Input: dimensioned drawing with shaded views. Units: mm. Origin: part minimum x, y, z. Round coordinates to 2 decimals unless told otherwise and drop trailing zeros. Order: outer loops, then holes, each group sorted by start corner. A loop starts at its lowest first (then second) coordinate and runs counter-clockwise, first axis right, second up. Notation, with made-up numbers: M -9,10 L 32,10 A10 ccw 32,27 Z; hole C -34.5,-18.5 d9. An arc over 180 degrees is marked long. Use one line per item in the form item = value. Start each with the question number.
Q1. Material intervals for probe 1 along Y at (x, z) = (128.5, 2.45); probe 2 along X at (y, z) = (38, 1.25); probe 3 along X at (y, z) = (9, 2.2), sorted ascending.
Q2. Section B-B (x = 63). Return the cut outline in (y, z).
Q3. Section C-C (z = 1.1). Return the cut outline in (x, y).
Q4. Section A-A (y = 65.5). Return the cut outline in (x, z), plus the area to 3 significant figures.
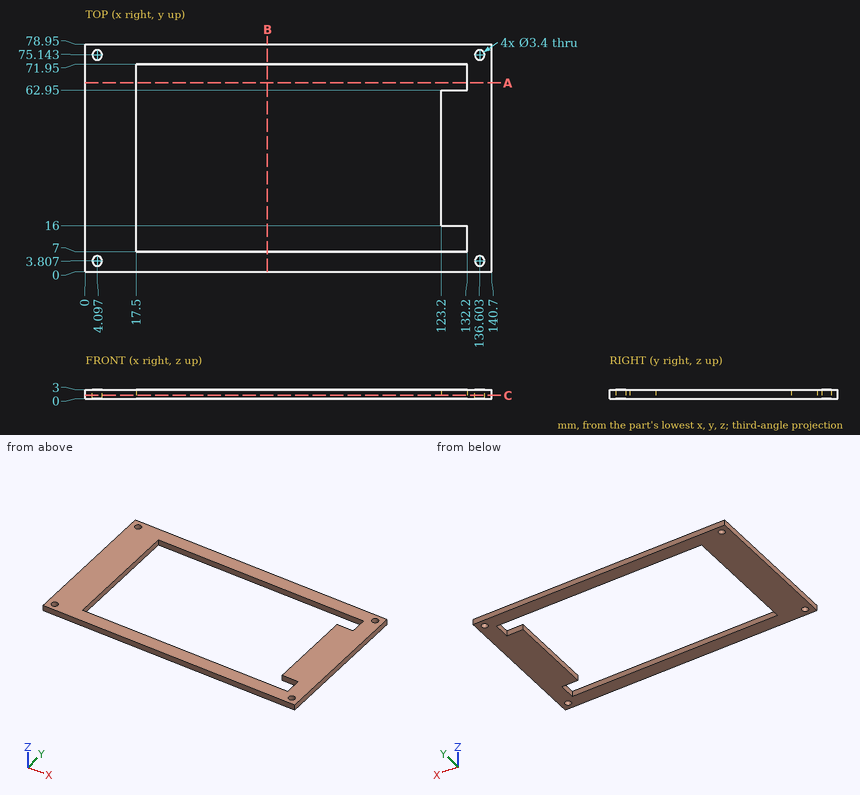
Results list:
q1.probe_1 = 0 to 7, 16 to 62.95, 71.95 to 78.95
q1.probe_2 = 0 to 17.5, 123.2 to 140.7
q1.probe_3 = 0 to 17.5, 132.2 to 140.7
q2.outline = M 0,0 L 7,0 L 7,3 L 0,3 Z; M 71.95,0 L 78.95,0 L 78.95,3 L 71.95,3 Z
q3.outline = M 0,0 L 140.7,0 L 140.7,78.95 L 0,78.95 Z; hole C 4.1,3.81 d3.4; hole C 4.1,75.14 d3.4; hole M 17.5,7 L 132.2,7 L 132.2,16 L 123.2,16 L 123.2,62.95 L 132.2,62.95 L 132.2,71.95 L 17.5,71.95 Z; hole C 136.6,3.81 d3.4; hole C 136.6,75.14 d3.4
q4.outline = M 0,0 L 17.5,0 L 17.5,3 L 0,3 Z; M 132.2,0 L 140.7,0 L 140.7,3 L 132.2,3 Z
q4.area = 78.0 mm2
